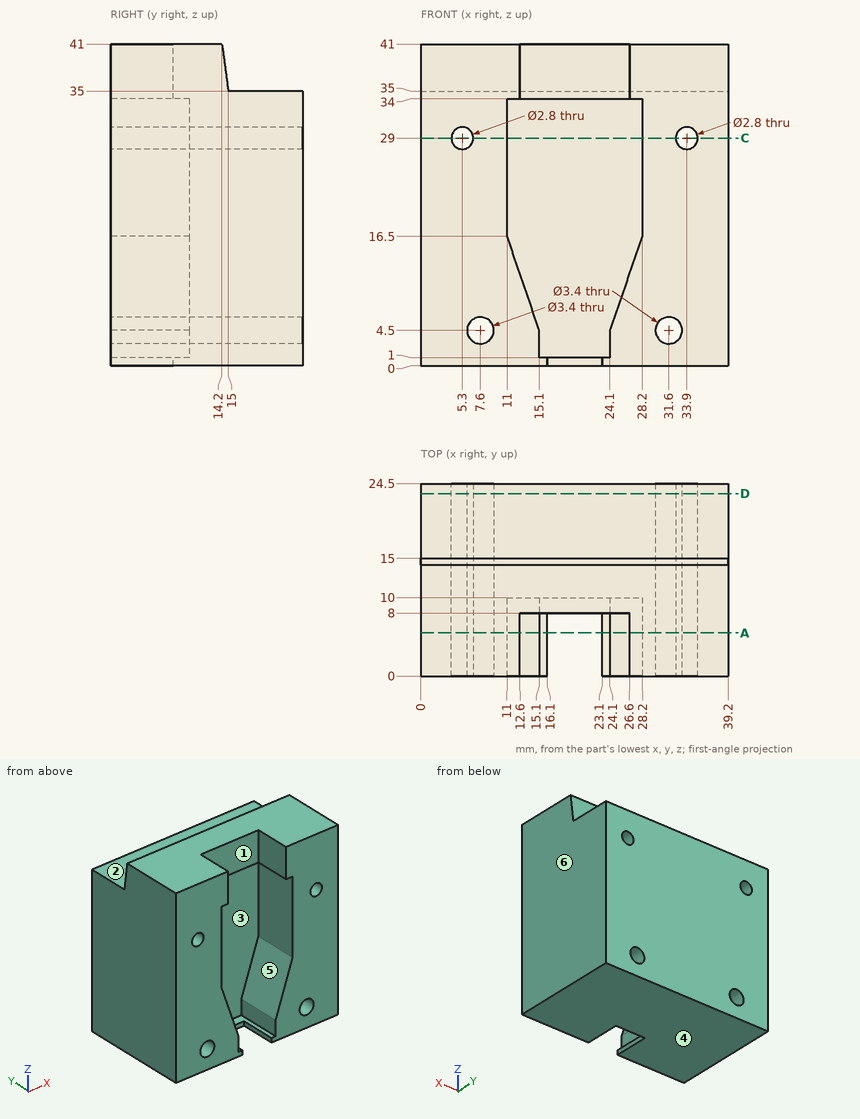
The figure shows three views and two pictorial views of one solid part (mm, origin at its lowest corner). Answer the questions. A direction names the side the tool comes from. Round coordinates to 2 decimals unless told otherwise and drop trailing zeros. Write each loop counter-clockwise with the first axis right and the second up, starting at its lowest first coordinate (ties: lowest second). Pieces come first, ordered by that corner, then holes. Notation, with made-up numbers: M 7,-35 L 19,-35 A34 cw 19,1 Z; hole C 23.5,34 d2. An arc over 180 degrees is marked long. Write each question's results on one line, items separated by ' | '. Start each with the question number.
(1) For the marked faces 1, 2 and 3, determine the directions among +Z, -Z, +X, -X, +Y, -Y from which every point of the face is accessible in a straight line to the end or side of a thin tool.
(2) The part is cut by section D-D, the plane y = 23.25. Write down the section's boundary in (x, z).
(3) Each of these flat-tipped pins is pushed along its axis until it touches: P1, Ø6, axis at y = 7.5, z = 5.5, coming from the -X side; P2, Ø7.5, axis at x = 21.5, z = 37, coming from the -Y side; P3, Ø2, axis at x = 15, z = 8, coming from the -Y side; P4, Ø5, axis at x = 20, y = 21, coming from the +Z side. Where does it stop, or does it pass through?
(4) Find the intervals of material crossed by line 1 (Z direction, x = 5.3, y = 13); line 2 (X direction, y = 5, z = 16.5); line 3 (X direction, y = 5.25, z = 29.5), in increasing order.
(5) The part is cut by section A-A, the plane y = 5.5. Write down the section's boundary in (x, z), and give its area (3 significant figures).
(6) The part is cut by section C-C, the plane z = 29. Write down the section's boundary in (x, y), and give its area (3 significant figures).
(7) Determine the mould class of the marked faces 4, 5 and 6 for opening direction Z: +Z half, -Z half, draft (parallel to the pull), parting line (faces both ways), or undercut.
Worked answers:
1) face 1: +Z, -Y | face 2: +Z, +X, -X, +Y | face 3: -Y
2) outline: M 0,0 L 39.2,0 L 39.2,35 L 0,35 Z; hole C 5.3,29 d2.8; hole C 7.6,4.5 d3.4; hole C 31.6,4.5 d3.4; hole C 33.9,29 d2.8
3) P1: stops at x = 0 | P2: stops at y = 8 | P3: stops at y = 10 | P4: stops at z = 35
4) line 1: z = 0 to 27.6, 30.4 to 41 | line 2: x = 0 to 11, 28.2 to 39.2 | line 3: x = 0 to 3.99, 6.61 to 11, 28.2 to 32.59, 35.21 to 39.2
5) outline: M 0,0 L 16.1,0 L 16.1,1 L 15.1,1 L 15.1,4.5 L 11,16.5 L 11,34 L 12.6,34 L 12.6,41 L 0,41 Z; M 23.1,0 L 39.2,0 L 39.2,41 L 26.6,41 L 26.6,34 L 28.2,34 L 28.2,16.5 L 24.1,4.5 L 24.1,1 L 23.1,1 Z; hole C 5.3,29 d2.8; hole C 7.6,4.5 d3.4; hole C 31.6,4.5 d3.4; hole C 33.9,29 d2.8 | area: 982 mm²
6) outline: M 0,0 L 3.9,0 L 3.9,24.5 L 0,24.5 Z; M 6.7,0 L 11,0 L 11,10 L 28.2,10 L 28.2,0 L 32.5,0 L 32.5,24.5 L 6.7,24.5 Z; M 35.3,0 L 39.2,0 L 39.2,24.5 L 35.3,24.5 Z | area: 651 mm²
7) face 4: -Z half | face 5: undercut | face 6: draft
